from build123d import *

# Parameters (mm, degrees)
BLANKSKE_W               = 20
BLANKSKE_H               = 5.5
BLANK_DEPTH              = 4
TOOTHCUTSIM_DEPTH        = 22.124630174
TEETHCUTS_COUNT          = 14
TEETHCUTS_PITCH          = 1.570796325
SKETCH1_W                = 2.5
SKETCH1_H                = 13
BOSS_EXTRUDE1_DEPTH      = 22
BOSS_EXTRUDE3_DEPTH      = 5
BOSS_EXTRUDE3_DEPTH_BACK = 34
SKETCH3_W                = 4
SKETCH3_H                = 4.375
CUT_EXTRUDE1_DEPTH       = 38.175260591
CUT_EXTRUDE1_DEPTH_BACK  = 38.175260591
SKETCH4_W                = 4.5
SKETCH4_H                = 8.625
FILLET1_R                = 3


with BuildPart() as part:
    # BlankSke → Blank (new body)
    with BuildSketch(Plane.XY):
        with Locations((10, 2.75)):
            Rectangle(BLANKSKE_W, BLANKSKE_H)
    extrude(amount=-BLANK_DEPTH)

    # TooCutSkeSim → ToothCutSim (cut, through all)
    with BuildSketch(Plane.XY):
        Polygon((0.222217685, 4.375), (-0.222217685, 4.375), (-0.640929042, 5.5254), (0.640929042, 5.5254), align=None)
    toothcutsim = extrude(amount=-TOOTHCUTSIM_DEPTH, mode=Mode.SUBTRACT)

    # TeethCuts: ToothCutSim ×14
    with Locations(*[(i * TEETHCUTS_PITCH, 0, 0) for i in range(1, TEETHCUTS_COUNT)]):
        add(toothcutsim, mode=Mode.SUBTRACT)

    # Sketch1 → Boss-Extrude1 (add)
    with BuildSketch(Plane.XY):
        with Locations((8.25, 6.5)):
            Rectangle(SKETCH1_W, SKETCH1_H)
    extrude(amount=BOSS_EXTRUDE1_DEPTH)

    # Sketch3 → Boss-Extrude3 (add, two sides: drawn at the far end of the back side and taken through both)
    with BuildSketch(Plane.ZY.offset(-BOSS_EXTRUDE3_DEPTH_BACK)):
        with Locations((-2, 2.1875)):
            Rectangle(SKETCH3_W, SKETCH3_H)
    extrude(amount=BOSS_EXTRUDE3_DEPTH + BOSS_EXTRUDE3_DEPTH_BACK)

    # Sketch4 → Cut-Extrude1 (cut, two sides: drawn at the far end of the back side and taken through both)
    with BuildSketch(Plane.ZY.offset(-7).offset(-CUT_EXTRUDE1_DEPTH_BACK)):
        with Locations((2.25, 8.6875)):
            Rectangle(SKETCH4_W, SKETCH4_H)
    extrude(amount=CUT_EXTRUDE1_DEPTH + CUT_EXTRUDE1_DEPTH_BACK, mode=Mode.SUBTRACT)

    # Fillet1
    # the kernel refuses this fillet: 3 mm, written as the material it adds along each edge
    with BuildSketch(Plane(origin=(7, 0, 0), x_dir=(0, 0, 1), z_dir=(0, 1, 0))) as fillet1_piece_1:
        with BuildLine():
            CenterArc((FILLET1_R, -FILLET1_R), FILLET1_R, 90, 90)
            Line((0, -FILLET1_R), (0, 0))
            Line((0, 0), (FILLET1_R, 0))
        make_face()
    extrude(amount=4.375)
    with BuildSketch(Plane(origin=(9.5, 0, 0), x_dir=(0, 0, 1), z_dir=(0, 1, 0))) as fillet1_piece_2:
        with BuildLine():
            CenterArc((FILLET1_R, FILLET1_R), FILLET1_R, 180, 90)
            Line((0, FILLET1_R), (0, 0))
            Line((0, 0), (FILLET1_R, 0))
        make_face()
    extrude(amount=4.375)
    with BuildSketch(Plane(origin=(9.5, -7.5, 0), x_dir=(0, 0, 1), z_dir=(0, 1, 0))) as fillet1_piece_3_section:
        with BuildLine():
            CenterArc((FILLET1_R, FILLET1_R), FILLET1_R, 180, 90)
            Line((0, FILLET1_R), (0, 0))
            Line((0, 0), (FILLET1_R, 0))
        make_face()
    fillet1_piece_3 = extrude(amount=19.375, mode=Mode.PRIVATE)
    fillet1_piece_3 = split(fillet1_piece_3, bisect_by=Plane(origin=(11.636487366, 4.375, 0.067590567), z_dir=(0, 1, 0)), keep=Keep.TOP, mode=Mode.PRIVATE)
    fillet1_piece_3 = split(fillet1_piece_3, bisect_by=Plane(origin=(11.636487366, 5.5, 0.067590567), z_dir=(0, -1, 0)), keep=Keep.TOP, mode=Mode.PRIVATE)
    fillet1_piece_3 = split(fillet1_piece_3, bisect_by=Plane(origin=(11.407964632, 4.897495122, 0.067590567), z_dir=(0.9396926207859105, -0.3420201433256629, 0)), keep=Keep.TOP, mode=Mode.PRIVATE)
    fillet1_piece_3 = split(fillet1_piece_3, bisect_by=Plane(origin=(12.120177158, 4.990368336, 0.067590567), z_dir=(-0.9396926207859105, -0.3420201433256629, 0)), keep=Keep.TOP, mode=Mode.PRIVATE)
    add(fillet1_piece_3)
    with BuildSketch(Plane(origin=(9.5, -7.5, 0), x_dir=(0, 0, 1), z_dir=(0, 1, 0))) as fillet1_piece_4_section:
        with BuildLine():
            CenterArc((FILLET1_R, FILLET1_R), FILLET1_R, 180, 90)
            Line((0, FILLET1_R), (0, 0))
            Line((0, 0), (FILLET1_R, 0))
        make_face()
    fillet1_piece_4 = extrude(amount=19.375, mode=Mode.PRIVATE)
    fillet1_piece_4 = split(fillet1_piece_4, bisect_by=Plane(origin=(10.146205087, 4.375, 0.590480104), z_dir=(0, 1, 0)), keep=Keep.TOP, mode=Mode.PRIVATE)
    fillet1_piece_4 = split(fillet1_piece_4, bisect_by=Plane(origin=(9.84999644, 4.932740127, 0.590480104), z_dir=(0.9396926207859105, -0.3420201433256629, 0)), keep=Keep.TOP, mode=Mode.PRIVATE)
    fillet1_piece_4 = split(fillet1_piece_4, bisect_by=Plane(origin=(10.146205087, 5.5, 0.590480104), z_dir=(0, -1, 0)), keep=Keep.TOP, mode=Mode.PRIVATE)
    fillet1_piece_4 = split(fillet1_piece_4, bisect_by=Plane(origin=(10.555389409, 4.97385991, 0.590480104), z_dir=(-0.9396926207859105, -0.3420201433256629, 0)), keep=Keep.TOP, mode=Mode.PRIVATE)
    add(fillet1_piece_4)


with BuildPart() as body_2:
    # Mirror1: mirrored copy
    add(part.part.mirror(Plane(origin=(34, 0, -4), x_dir=(0, 0, 1), z_dir=(1, 0, 0))))


solid = body_2.part
Input: part model. Units: mm. Frame: model coordinates. A direction names the side the tool comes from. Give positions to 0.01 mm unless a question says otherwise; leave off trailing zeros. Loops run counter-clockwise (first coordinate to the right, second up) from the corner with the lowest first, then second, coordinate; pieces in that order, holes last. Notation, with made-up numbers: (58.5, 85.5) -> (65.5, 85.5) arc R37 cw to (65.5, 122.5) -> close; hole circle Ø8 at (-18, -4). An arc over 180 degrees is marked (long way). Answer as a JSON object with one key per item and string values. Group by question number.
Item 1: Cut plane A-A, the plane y = 1.25. Return the cut outline in (x, z).
Item 2: Line query: probe 1 along X at (y, z) = (10.75, 19.5); probe 2 along Y at (x, z) = (49, -2.25) (3 decimals); probe 3 along Y at (x, z) = (53, -0.5). Output: solid intervals per line, ascending.
Item 3: Pull-direction query (X, two-part tool) for faces 1 (the flat face through (61, 6, 12)), 2 (the flat face through (54.287, 4.93, -1.972)), 3 (the flat face through (41, 4.375, -2)); classes: released by +X, released by -X, zero draft, split by the parting line, or undercut.
Item 4: Reachability of faces 4 (the flat face through (59, 4.93, -1.97)), 5 (the flat face through (58.5, 6, 12)), 6 (the flat face through (53.43, 4.95, -1.97)) from +Z, -Z, +X, -X, +Y, -Y: full face, straight path, thin tool, end or side. Return the list, or none.
Item 5: Pin query (flat end, axial travel): P1, Ø4.5, axis at x = 71.5, z = -2.5, coming from the +Y side (3 decimals); P2, Ø1.6, axis at x = 48, y = 4, coming from the +Z side; P3, Ø6, axis at x = 54.5, y = 6, coming from the -Z side; P4, Ø2, axis at x = 60, y = 8.5, coming from the -Z side. Return the tip coordinate at first contact, or that it passes through.
Item 6: Cut plane B-B, the plane z = 20. Return the cut outline in (x, y), and give its area (3 significant figures).
Item 7: Cut plane C-C, the plane x = 69.5. Return the cut outline in (y, z) (3 decimals).
Checks:
{
 "1": {"outline": "(34, -4) -> (73, -4) -> (73, 0) -> (64, 0) arc R3 cw to (61, 3) -> (61, 22) -> (58.5, 22) -> (58.5, 3) arc R3 cw to (55.5, 0) -> (34, 0) -> close"},
 "2": {"probe 1": "x = 58.5 to 61", "probe 2": "y = 0 to 4.375", "probe 3": "y = 0 to 5.5"},
 "3": {"face 1": "released by +X", "face 2": "undercut", "face 3": "zero draft"},
 "4": {"face 4": "-Z, +Y", "face 5": "+Z, -X, +Y, -Y", "face 6": "+Z, -Z, +Y"},
 "5": {"P1": "stops at y = 4.375", "P2": "stops at z = 0", "P3": "stops at z = -4", "P4": "stops at z = 4.5"},
 "6": {"outline": "(58.5, 0) -> (61, 0) -> (61, 13) -> (58.5, 13) -> close", "area": "32.5 mm²"},
 "7": {"outline": "(0, -4) -> (4.375, -4) -> (4.375, 0) -> (0, 0) -> close"}
}
